Answer from the drawing. Dimensions are ordinates in mm from the lowest x, y and z of the part. Coordinates: 2 decimals unless noted, no trailing zeros. Write each loop counter-clockwise with the first axis right and the second up, starting at its lowest first coordinate (ties: lowest second). Pieces come first, ordered by that corner, then holes.
(1) Find the intervals of material crossed by probe 1 along Z at (x, y) = (7.25, 0.15); probe 2 along Z at (x, y) = (9.75, 1.85); probe 3 along X at (y, z) = (0.65, 7.5), in increasing order.
(2) Given pin 1 (3 mm diameter, centred on x = 7.5, z = 157.5, fed in from +Y), flat-ended and moving along its own axis, determine where the tip first touches the part or whether it passes through.
(3) Section A-A on y = 0.6 is taken. Write down the section's boundary in (x, z), then the cut area to 3 significant figures.
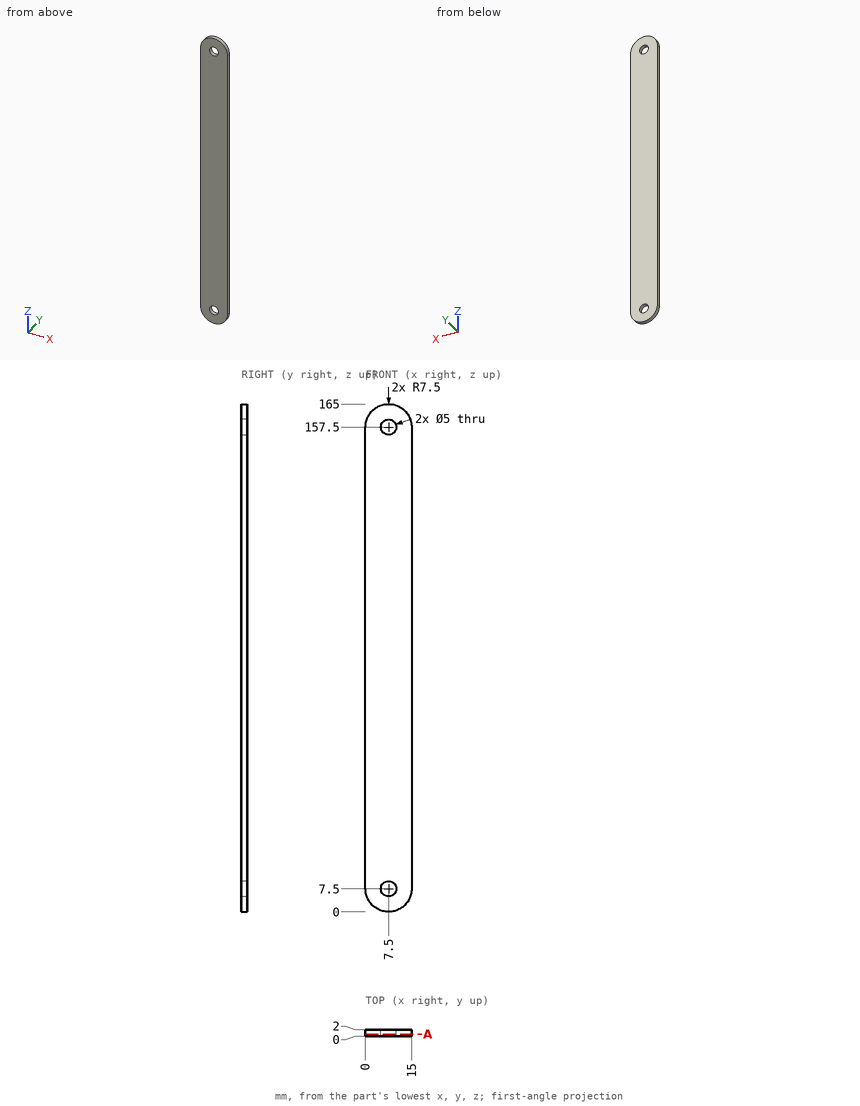
Response:
1. probe 1: z = 0 to 5.01, 9.99 to 155.01, 159.99 to 165
1. probe 2: z = 0.35 to 6.41, 8.59 to 156.41, 158.59 to 164.65
1. probe 3: x = 0 to 5, 10 to 15
2. pin 1: passes through
3. outline: (0, 7.5) arc R7.5 ccw to (15, 7.5) - (15, 157.5) arc R7.5 ccw to (0, 157.5) - close; hole circle Ø5 at (7.5, 7.5); hole circle Ø5 at (7.5, 157.5)
3. area: 2,390 mm2
